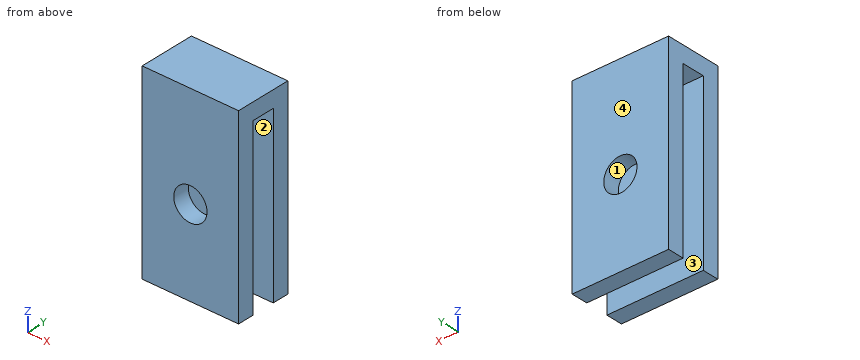
```python
from build123d import *

# Parameters (mm, degrees)
SKETCH1_W           = 14.732
SKETCH1_H           = 26.416
SKETCH1_R           = 2.54
BOSS_EXTRUDE1_DEPTH = 8.5979
SKETCH2_W           = 14.732
SKETCH2_H           = 8.5979
BOSS_EXTRUDE2_DEPTH = 2.54
SKETCH3_W           = 26.416
SKETCH3_H           = 3.5179
CUT_EXTRUDE1_DEPTH  = 25.4


with BuildPart() as part:
    # Sketch1 → Boss-Extrude1 (new body)
    with BuildSketch(Plane(origin=(0, 0, 0), x_dir=(1, 0, 0), z_dir=(0, 1, 0))):
        with Locations((7.366, 13.208)):
            Rectangle(SKETCH1_W, SKETCH1_H)
        with Locations(Location((7.366, 13.208, 0), (0, 0, 270))):
            Circle(SKETCH1_R, mode=Mode.SUBTRACT)
    extrude(amount=BOSS_EXTRUDE1_DEPTH)

    # Sketch2 → Boss-Extrude2 (add)
    with BuildSketch(Plane.XY):
        with Locations((7.366, 4.29895)):
            Rectangle(SKETCH2_W, SKETCH2_H)
    extrude(amount=BOSS_EXTRUDE2_DEPTH)

    # Sketch3 → Cut-Extrude1 (cut)
    with BuildSketch(Plane(origin=(14.732, 0, 0), x_dir=(0, 0, -1), z_dir=(1, 0, 0))):
        with Locations((13.208, 4.29895)):
            Rectangle(SKETCH3_W, SKETCH3_H)
    extrude(amount=-CUT_EXTRUDE1_DEPTH, mode=Mode.SUBTRACT)


solid = part.part
```
The model under review builds one solid part; all positions refer to its coordinate system, in mm. Face numbers are marked on the shaded views. Coordinates: 2 decimals unless noted, no trailing zeros. Write each loop counter-clockwise with the first axis right and the second up, starting at its lowest first coordinate (ties: lowest second). Pieces come first, ordered by that corner, then holes. Notation, with made-up numbers: (2, 2) - (48, 2) arc R22 cw to (48, 22) - close; hole circle Ø8 at (56.25, 9). An arc over 180 degrees is marked (long way). Answer in a Markdown table with one row per item. Add a question column.
Q1. Consider section A-A on z = -1. Give the boundary of the cut face in (x, y), then the cut area to 3 significant figures.
Q2. To check wall thickness, follow line 1 along Y through (x, z) = (6.75, -18.5); line 2 along Z through (x, y) = (10.5, 5.75); line 3 along X through (y, z) = (6.25, -15.25). State the ranges of each line that lie inside material, in increasing order. Write a range as from..to.
Q3. Consider section B-B on x = 9.5. Give the boundary of the cut face in (y, z).
Q4. Consider section D-D on x = 4. Give the boundary of the cut face in (y, z), then the cut area to 3 significant figures.
Q5. Draft analysis for pull direction Y (two halves, no side actions). For the marked faces 1, 2, 3 and 4, state which applies: +Y half, -Y half, draft (parallel to the pull), parting line (faces both ways), or undercut.
Q6. Clearance check with a flat-ended pin moving along its axis: pin 1 (1.8 mm diameter, centred on x = 10.5, y = 4, fed in from -Z). State where the tip first meets the part, or that it passes through.
Q7. Consider section C-C on z = -11. Give the boundary of the cut face in (x, y).
Answers below:
| question | item | result |
|---|---|---|
| 1 | outline | (0, 0) - (14.73, 0) - (14.73, 2.54) - (0, 2.54) - close; (0, 6.06) - (14.73, 6.06) - (14.73, 8.6) - (0, 8.6) - close |
| 1 | area | 74.8 mm² |
| 2 | line 1 | 0..2.54, 6.06..8.6 |
| 2 | line 2 | 0..2.54 |
| 2 | line 3 | 0..5.86, 8.88..14.73 |
| 3 | outline | (0, -26.42) - (2.54, -26.42) - (2.54, -14.59) - (0, -14.59) - close; (0, -11.83) - (2.54, -11.83) - (2.54, 0) - (6.06, 0) - (6.06, -11.83) - (8.6, -11.83) - (8.6, 2.54) - (0, 2.54) - close; (6.06, -26.42) - (8.6, -26.42) - (8.6, -14.59) - (6.06, -14.59) - close |
| 4 | outline | (0, -26.42) - (2.54, -26.42) - (2.54, 0) - (6.06, 0) - (6.06, -26.42) - (8.6, -26.42) - (8.6, 2.54) - (0, 2.54) - close |
| 4 | area | 156 mm² |
| 5 | face 1 | draft |
| 5 | face 2 | undercut |
| 5 | face 3 | undercut |
| 5 | face 4 | +Y half |
| 6 | pin 1 | z = 0 |
| 7 | outline | (0, 0) - (6.11, 0) - (6.11, 2.54) - (0, 2.54) - close; (0, 6.06) - (6.11, 6.06) - (6.11, 8.6) - (0, 8.6) - close; (8.62, 0) - (14.73, 0) - (14.73, 2.54) - (8.62, 2.54) - close; (8.62, 6.06) - (14.73, 6.06) - (14.73, 8.6) - (8.62, 8.6) - close |
